```python
from build123d import *

# Parameters (mm, degrees)
BOSS_EXTRUDE1_DEPTH = 2
SKETCH2_R           = 0.85
BOSS_EXTRUDE2_DEPTH = 10.2
FILLET1_R           = 3


with BuildPart() as part:
    # Sketch1 → Boss-Extrude1 (new body)
    with BuildSketch(Plane.XY):
        with BuildLine():
            Line((-7.01, 5.520677243), (-2.014670258, 2.636622271))
            Line((-2.014670258, 2.636622271), (5.62, 7.0445012))
            ThreePointArc((5.62, 7.0445012), (7.669038106, 6.495463094), (7.12, 4.446424988))
            Line((7.12, 4.446424988), (-0.514670258, 0.03854606))
            ThreePointArc((-0.514670258, 0.03854606), (-2.014670258, -0.363377729), (-3.514670258, 0.03854606))
            Line((-3.514670258, 0.03854606), (-8.51, 2.922601032))
            ThreePointArc((-8.51, 2.922601032), (-9.059038106, 4.971639137), (-7.01, 5.520677243))
        make_face()
        with BuildLine():
            Line((-7.640528879, 4.441244809), (-5.883683502, 3.48547584))
            ThreePointArc((-5.883683502, 3.48547584), (-5.783548951, 3.146399047), (-6.122625744, 3.046264496))
            Line((-6.122625744, 3.046264496), (-7.879471121, 4.002033465))
            ThreePointArc((-7.879471121, 4.002033465), (-7.979605672, 4.341110258), (-7.640528879, 4.441244809))
        make_face(mode=Mode.SUBTRACT)
    boss_extrude1 = extrude(amount=BOSS_EXTRUDE1_DEPTH)

    # Sketch2 → Boss-Extrude2 (add)
    with BuildSketch(Plane.XY.offset(2)):
        with Locations((6.37, 5.745463094)):
            Circle(SKETCH2_R)
    extrude(amount=BOSS_EXTRUDE2_DEPTH)

    # Mirror1: Boss-Extrude1 across plane
    add(boss_extrude1.mirror(Plane.XY.offset(7.1)))

    # Fillet1
    fillet1_edges = [part.edges().sort_by_distance(p)[0] for p in [
        (-2.014670258, 2.636622271, 1),
        (-2.014670258, 2.636622271, 13.2),
    ]]
    fillet(fillet1_edges, radius=FILLET1_R)


solid = part.part
```
Can you work these out from the model? Positions are in its coordinate system, mm. A direction names the side the tool comes from. Coordinates: 2 decimals unless noted, no trailing zeros. Order: outer loops, then holes, each group sorted by start corner. A loop starts at its lowest first (then second) coordinate and runs counter-clockwise, first axis right, second up. Notation, with made-up numbers: (-22, 3.25) - (-3, 3.25) arc R16 cw to (-3, 15.25) - close; hole circle Ø7 at (12, -28.75). An arc over 180 degrees is marked (long way). Answer in a Markdown table with one row per item.
1. Suppose I cut it at A-A (z = 1.75). Please give me the cut outline in (x, y).
Reply:
| item | result |
|---|---|
| outline | (-8.51, 2.92) - (-3.51, 0.04) arc R3 ccw to (-0.51, 0.04) - (7.12, 4.45) arc R1.5 ccw to (5.62, 7.04) - (-0.51, 3.5) arc R3 cw to (-3.51, 3.5) - (-7.01, 5.52) arc R1.5 ccw to start; hole (-7.88, 4) - (-6.12, 3.05) arc R0.25 ccw to (-5.88, 3.49) - (-7.64, 4.44) arc R0.25 ccw to start |
2. If we mould it in two halves opening along Z, with no side actions, what happens to faces 1 (the flat face through (-1, 3, 0)), 2 (the flat face through (-5.287, 4.526, 13.214)), 3 (the flat face through (-1, 3, 12.2))? For each: pulls with the +Z half, pulls with the -Z half, needs draft (parallel to the pull), parting line crosses it, or undercut.
Reply:
| item | result |
|---|---|
| face 1 | pulls with the -Z half |
| face 2 | needs draft |
| face 3 | undercut |
3. For faces 4 (the flat face through (-5.287, 4.526, 0.986)), 5 (the flat face through (-1, 3, 14.2)), 6 (the flat face through (-6.99, 3.52, 13.21)), which set-ups out of +Z, -Z, +X, -X, +Y, -Y let a thin tool reach every point of the face, with its end or its side?
Reply:
| item | result |
|---|---|
| face 4 | +Z, -Z, +Y |
| face 5 | +Z, +X, -X, +Y, -Y |
| face 6 | +Z, -Z |
4. Suppose I cut it at C-C (x = -3.75). Please give me the cut outline in (y, z).
Reply:
| item | result |
|---|---|
| outline | (0.17, 0) - (3.64, 0) - (3.64, 2) - (0.17, 2) - close; (0.17, 12.2) - (3.64, 12.2) - (3.64, 14.2) - (0.17, 14.2) - close |
5. Suppose I cut it at D-D (x = 6.37). Please give me the cut outline in (y, z), and give its area (3 significant figures).
Reply:
| item | result |
|---|---|
| outline | (4.01, 0) - (7.25, 0) - (7.25, 2) - (6.6, 2) - (6.6, 12.2) - (7.25, 12.2) - (7.25, 14.2) - (4.01, 14.2) - (4.01, 12.2) - (4.9, 12.2) - (4.9, 2) - (4.01, 2) - close |
| area | 30.3 mm^2 |
6. Suppose I cut it at B-B (y = 2.25). Please give me the cut outline in (x, z), and give its area (3 significant figures).
Reply:
| item | result |
|---|---|
| outline | (-7.35, 0) - (3.32, 0) - (3.32, 2) - (-7.35, 2) - close; (-7.35, 12.2) - (3.32, 12.2) - (3.32, 14.2) - (-7.35, 14.2) - close |
| area | 42.6 mm^2 |
7. If I drill on line 1 along Z through (x, y) = (2.25, 5); line 2 along Y through (x, z) = (-1.25, 1.5); line 3 along X through (y, z) = (1.5, 12.25), over which ranges is the centre line in solid material (lowest first)?
Reply:
| item | result |
|---|---|
| line 1 | z = 0 to 2, 12.2 to 14.2 |
| line 2 | y = -0.26 to 3.2 |
| line 3 | x = -6.05 to 2.02 |
8. For pin 1 (5 mm diameter, centred on x = 4, z = 7.5, fed in from +Y), with a flat end and sliding along its axis, tell me the tip position at first contact or that it passes through.
Reply:
| item | result |
|---|---|
| pin 1 | stops at y = 6.6 |
